Geometry check sheet. Reference: the model listing, model coordinates, mm. A direction names the side the tool comes from. Coordinates: 2 decimals unless noted, no trailing zeros. Order: outer loops, then holes, each group sorted by start corner. A loop starts at its lowest first (then second) coordinate and runs counter-clockwise, first axis right, second up. Notation, with made-up numbers: (49, 63) - (67, 63) arc R18 ccw to (67, 98) - close; hole circle Ø1 at (42.5, -0.75). An arc over 180 degrees is marked (long way). Return JSON: item names as keys, results as strings. Group by question number.
Item 1: Section check D-D on y = 1. Enter the section's corners in (x, z), then the cut area to 3 significant figures.
Item 2: Section check A-A on x = 8. Enter the section's corners in (y, z).
Item 3: Section check C-C on x = -1. Enter the section's corners in (y, z), then the cut area to 3 significant figures.
Item 4: Gauge pin test, flat ends, axial feed: pin 1 (6 mm diameter, centred on x = -5, y = 3, fed in from +Z); pin 2 (0.7 mm diameter, centred on y = 9, z = 1.5, fed in from +X); pin 3 (0.6 mm diameter, centred on y = 8.5, z = 0, fed in from +X); pin 4 (5 mm diameter, centred on x = 5, y = 11, fed in from +Z). Record the tip position at first contact, or that the pin passes through.
Item 5: Section check B-B on z = 0. Enter the section's corners in (x, y), then the cut area to 3 significant figures.
Item 6: Tool access check on faces 1 (the flat face through (-7, -12.267, 0)), 2 (the flat face through (4.9, -9, 1)), 3 (the flat face through (7, 12.267, 0)). Record the directions out of +Z, -Z, +X, -X, +Y, -Y that give a thin tool (end or side, any length) a straight path to the whole face; none if there is none.
Item 7: Scan lines: probe 1 along Y at (x, z) = (9.25, 0.05); probe 2 along Y at (x, z) = (4.25, 1.5); probe 3 along Y at (x, z) = (0.25, 0.95). Record each from-to range of solid material in increasing order.
Item 8: Draft check along Y on faces 4 (the cylindrical face through (-0.069, 9.315, 1.274)), 5 (the flat face through (-5, -10, 0)), 6 (the flat face through (-10, 0, 0)), 7 (the flat face through (0, 17, 0)). Enter one of: pulls with the +Y half, pulls with the -Y half, needs draft (parallel to the pull), parting line crosses it, or undercut.
from build123d import *

# Parameters (mm, degrees)
F1_DEPTH = 0.6
F2_R     = 0.5
F3_DEPTH = 4.9


with BuildPart() as f1:
    # F0 (on Top) → F1 (new body, symmetric)
    with BuildSketch(Plane.XY):
        Polygon((10, 12.267178), (10, 17), (-10, 17), (-10, 12.267178), (-5, 12.267178), (-5, 7.267178), (-10, 7.267178), (-10, -7.267178), (-5, -7.267178), (-5, -12.267178), (-10, -12.267178), (-10, -17), (10, -17), (10, -12.267178), (5, -12.267178), (5, -7.267178), (10, -7.267178), (10, 7.267178), (5, 7.267178), (5, 12.267178), align=None)
    extrude(amount=F1_DEPTH, both=True)

    # F2 (on Right) → F3 (join, symmetric)
    with BuildSketch(Plane.YZ):
        with BuildLine():
            Line((-12.487299, 0.57844), (-7.044992, 0.55921))
            ThreePointArc((-7.044992, 0.55921), (-9.761185, 1.972687), (-12.487299, 0.57844))
        make_face()
        with Locations((-9.814223, 1.251517)):
            Circle(F2_R, mode=Mode.SUBTRACT)
        with BuildLine():
            ThreePointArc((12.487299, 0.57844), (9.761185, 1.972687), (7.044992, 0.55921))
            Line((7.044992, 0.55921), (12.487299, 0.57844))
        make_face()
        with Locations((9.814223, 1.251517)):
            Circle(F2_R, mode=Mode.SUBTRACT)
    extrude(amount=F3_DEPTH, both=True)


solid = f1.part
Computed:
{
 "1": {"outline": "(-10, -0.6) - (10, -0.6) - (10, 0.6) - (-10, 0.6) - close", "area": "24.0 mm²"},
 "2": {"outline": "(-17, -0.6) - (-12.27, -0.6) - (-12.27, 0.6) - (-17, 0.6) - close; (-7.27, -0.6) - (7.27, -0.6) - (7.27, 0.6) - (-7.27, 0.6) - close; (12.27, -0.6) - (17, -0.6) - (17, 0.6) - (12.27, 0.6) - close"},
 "3": {"outline": "(-17, -0.6) - (17, -0.6) - (17, 0.6) - (12.47, 0.6) arc R3.34 ccw to (7.07, 0.6) - (-7.07, 0.6) arc R3.34 ccw to (-12.47, 0.6) - (-17, 0.6) - close; hole circle Ø1 at (-9.81, 1.25); hole circle Ø1 at (9.81, 1.25)", "area": "49.6 mm²"},
 "4": {"pin 1": "stops at z = 0.6", "pin 2": "stops at x = 4.9", "pin 3": "stops at x = 5", "pin 4": "stops at z = 1.97"},
 "5": {"outline": "(-10, -17) - (10, -17) - (10, -12.27) - (5, -12.27) - (5, -7.27) - (10, -7.27) - (10, 7.27) - (5, 7.27) - (5, 12.27) - (10, 12.27) - (10, 17) - (-10, 17) - (-10, 12.27) - (-5, 12.27) - (-5, 7.27) - (-10, 7.27) - (-10, -7.27) - (-5, -7.27) - (-5, -12.27) - (-10, -12.27) - close", "area": "580 mm²"},
 "6": {"face 1": "+Z, -Z, -X", "face 2": "+Z, +X, +Y, -Y", "face 3": "+Z, -Z, +X"},
 "7": {"probe 1": "y = -17 to -12.27, -7.27 to 7.27, 12.27 to 17", "probe 2": "y = -11.49 to -10.25, -9.38 to -8.06, 8.06 to 9.38, 10.25 to 11.49", "probe 3": "y = -12.18 to -10.21, -9.42 to -7.37, 7.37 to 9.42, 10.21 to 12.18"},
 "8": {"face 4": "undercut", "face 5": "undercut", "face 6": "needs draft", "face 7": "pulls with the +Y half"}
}
